```python
from build123d import *

# Parameters (mm, degrees)
SKETCH1_W           = 11
SKETCH1_H           = 6
BOSS_EXTRUDE1_DEPTH = 5
SKETCH2_R           = 3
SKETCH2_R_2         = 1.9
BOSS_EXTRUDE2_DEPTH = 2.9
BOSS_EXTRUDE3_DEPTH = 2.9


with BuildPart() as part:
    # Sketch1 → Boss-Extrude1 (new body)
    with BuildSketch(Plane.XY):
        Rectangle(SKETCH1_W, SKETCH1_H)
    extrude(amount=BOSS_EXTRUDE1_DEPTH)

    # Sketch2 → Boss-Extrude2 (add)
    with BuildSketch(Plane(origin=(5.5, 0, 0), x_dir=(0, 0, -1), z_dir=(1, 0, 0))):
        with Locations(Location((-2.5, 0, 0), (0, 0, 90))):
            Circle(SKETCH2_R)
        with Locations(Location((-2.5, 0, 0), (0, 0, 90))):
            Circle(SKETCH2_R_2, mode=Mode.SUBTRACT)
    extrude(amount=BOSS_EXTRUDE2_DEPTH)

    # Sketch3 → Boss-Extrude3 (add)
    with BuildSketch(Plane(origin=(0, 0, 0), x_dir=(-1, 0, 0), z_dir=(0, 0, -1))):
        with BuildLine():
            Line((-3.6, 2.1), (-2.8, 2.1))
            ThreePointArc((-2.8, 2.1), (-2.7, 2), (-2.8, 1.9))
            Line((-2.8, 1.9), (-3.6, 1.9))
            ThreePointArc((-3.6, 1.9), (-3.7, 2), (-3.6, 2.1))
        make_face()
        with BuildLine():
            Line((3.9, 1.9), (3.1, 1.9))
            ThreePointArc((3.1, 1.9), (3, 2), (3.1, 2.1))
            Line((3.1, 2.1), (3.9, 2.1))
            ThreePointArc((3.9, 2.1), (4, 2), (3.9, 1.9))
        make_face()
        with BuildLine():
            Line((-1.7, -1.9), (-0.9, -1.9))
            ThreePointArc((-0.9, -1.9), (-0.8, -2), (-0.9, -2.1))
            Line((-0.9, -2.1), (-1.7, -2.1))
            ThreePointArc((-1.7, -2.1), (-1.8, -2), (-1.7, -1.9))
        make_face()
    extrude(amount=BOSS_EXTRUDE3_DEPTH)


solid = part.part
```
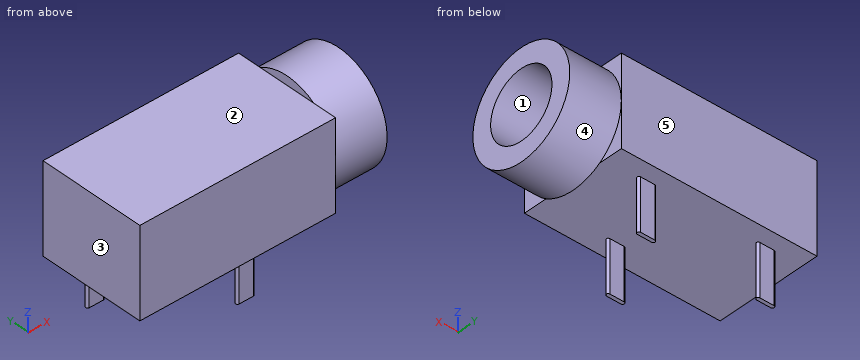
Geometry: final body of the model. Coordinates: model frame, mm. Face numbers are marked on the shaded views. A direction names the side the tool comes from. Give positions to 0.01 mm unless a question says otherwise; leave off trailing zeros. Loops run counter-clockwise (first coordinate to the right, second up) from the corner with the lowest first, then second, coordinate; pieces in that order, holes last. Notation, with made-up numbers: (42, 22.5) -> (60, 22.5) arc R15 ccw to (60, 43.5) -> close; hole circle Ø7 at (9, -21). An arc over 180 degrees is marked (long way). Use one line per item in the form item = value.
Item 1: Draft query along Z for the marked faces 1, 2 and 3. Return one class per face: pulls with the +Z half, pulls with the -Z half, needs draft (parallel to the pull), parting line crosses it, or undercut.
A:
face_1 = undercut
face_2 = pulls with the +Z half
face_3 = needs draft
Item 2: Access query for the marked faces 4 and 5. Directions: +Z, -Z, +X, -X, +Y, -Y. A direction counts if a zero-diameter tool reaches every point of the face in a straight line with its end or side. Return the directions, or none.
A:
face_4 = +X
face_5 = +Z, -Z, +X, -X, +Y
Item 3: Section query B-B on y = 0. Output: boundary loops of the cut face in (x, z), and give its area (3 significant figures).
A:
outline = (-5.5, 0) -> (5.5, 0) -> (5.5, -0.5) -> (8.4, -0.5) -> (8.4, 0.6) -> (5.5, 0.6) -> (5.5, 4.4) -> (8.4, 4.4) -> (8.4, 5.5) -> (5.5, 5.5) -> (5.5, 5) -> (-5.5, 5) -> close
area = 61.4 mm^2
Item 4: Section query A-A on z = -1.5. Output: boundary loops of the cut face in (x, y).
A:
outline = (-3.9, 1.9) -> (-3.1, 1.9) arc R0.1 ccw to (-3.1, 2.1) -> (-3.9, 2.1) arc R0.1 ccw to start; (0.9, -2.1) -> (1.7, -2.1) arc R0.1 ccw to (1.7, -1.9) -> (0.9, -1.9) arc R0.1 ccw to start; (2.8, 1.9) -> (3.6, 1.9) arc R0.1 ccw to (3.6, 2.1) -> (2.8, 2.1) arc R0.1 ccw to start
Item 5: Line query: probe 1 along Z at (x, y) = (6.55, 0); probe 2 along X at (y, z) = (1.4, 1.5); probe 3 along Z at (x, y) = (-3.5, -2.45). Output: solid intervals per line, ascending.
A:
probe_1 = -0.5 to 0.6, 4.4 to 5.5
probe_2 = -5.5 to 5.5
probe_3 = 0 to 5
Item 6: Pin query (flat end, axial travel): P1, Ø1.1, axis at y = -0.5, z = 2.5, coming from the +X side; P2, Ø5, axis at x = -0.5, z = -1, coming from the +Y side; P3, Ø0.9, axis at x = 3, z = -2, coming from the +Y side. Return the tip coordinate at first contact, or that it passes through.
A:
P1 = 5.5
P2 = 3
P3 = 2.1
Item 7: Section query D-D on z = 3.25. Output: boundary loops of the cut face in (x, y).
A:
outline = (-5.5, -3) -> (5.5, -3) -> (5.5, -2.9) -> (8.4, -2.9) -> (8.4, -1.75) -> (5.5, -1.75) -> (5.5, 1.75) -> (8.4, 1.75) -> (8.4, 2.9) -> (5.5, 2.9) -> (5.5, 3) -> (-5.5, 3) -> close
Item 8: Section query C-C on x = 3.25. Output: boundary loops of the cut face in (y, z).
A:
outline = (-3, 0) -> (1.9, 0) -> (1.9, -2.9) -> (2.1, -2.9) -> (2.1, 0) -> (3, 0) -> (3, 5) -> (-3, 5) -> close
